Check sheet for the modelled part. Datum: model origin and axes. Units: mm. Face numbers are marked on the shaded views. A direction names the side the tool comes from. Coordinates: 2 decimals unless noted, no trailing zeros. Order: outer loops, then holes, each group sorted by start corner. A loop starts at its lowest first (then second) coordinate and runs counter-clockwise, first axis right, second up.
1. Cross-section at B-B (x = -7.75). Enter the section's corners in (y, z).
2. Thickness scan on line 1 (Y direction, x = -20.45, z = 11.5); line 2 (X direction, y = 1, z = 10) (3 decimals); line 3 (Y direction, x = -13.5, z = 6.75). Record the ranges inside material, lowest first.
3. Set-up check for the marked faces 1, 2, 3, 4 and 5: record each of +Z, -Z, +X, -X, +Y, -Y from which the full face is reachable in a straight line by a thin tool's end or side.
4. Gauge pin test, flat ends, axial feed: pin 1 Ø1.8 at (y, z) = (2.5, 8) entering from +X; pin 2 Ø9 at (y, z) = (-8.5, 13.5) entering from +X; pin 3 Ø3 at (x, y) = (-12.5, -1) entering from -Z; pin 4 Ø1.2 at (y, z) = (3, 3.1) entering from -X. Record the tip position at first contact, or that the pin passes through.
5. Cross-section at C-C (y = 1.25). Enter the section's corners in (x, z), then the cut area to 3 significant figures.
6. Cross-section at D-D (x = -5.5). Enter the section's corners in (y, z).
7. Draft check along X on the marked faces 6, 7, 8 and 9. Enter one of: released by +X, released by -X, zero draft, split by the parting line, or undercut.
8. Cross-section at A-A (z = 10). Enter the section's corners in (x, y).
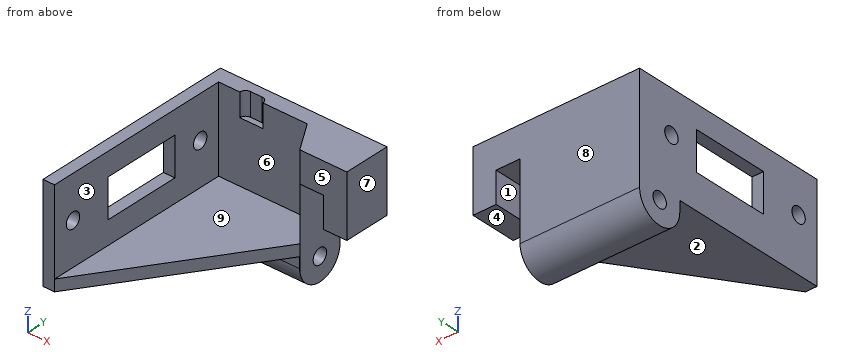
Autodesk Inventor part; units mm, degrees
ref_plane "YZ Plane" through (0, 0, 0) normal (1, 0, 0) x (0, 1, 0)
ref_plane "XZ Plane" through (0, 0, 0) normal (0, 1, 0) x (-1, 0, 0)
ref_plane "XY Plane" through (0, 0, 0) normal (0, 0, 1) x (1, 0, 0)
sketch "Sketch1" plane through (0, 0, 0) normal (0, 1, 0) x (-1, 0, 0)
  line L0 (0, 0) -> (21.6, 0)
  line L1 (21.6, 0) -> (21.6, 17)
  line L2 (21.6, 17) -> (0, 17)
  line L3 (0, 17) -> (0, 0)
  line L4 (6.1, 13) -> (3, 13)
  line L5 (3, 13) -> (3, 0)
  line L6 (3, 0) -> (6.1, 0)
  line L7 (6.1, 0) -> (6.1, 13)
  line L8 (21.6, 17) -> (9.1, 17)
  line L9 (9.1, 17) -> (9.1, 0)
  line L10 (9.1, 0) -> (21.6, 0)
  line L11 (21.6, 0) -> (21.6, 17)
  line L12 (9.1, 17) -> (21.6, 6.2)
  point P0 (21.6, 6.2)
  point P1 (9.1, 17)
  dimension "d1" = 17
  dimension "d2" = 3.1
  dimension "d3" = 3
  dimension "d4" = 3
  dimension "d5" = 6.2
  dimension "d17" = 13
  dimension "d18" = 12.5
extrude "Extrusion1" add sketch "Sketch1" along normal blind 6 contours L3 L2 L9 L0 L7 L4 L5 | L12 L1 L0 L9
sketch "Sketch2" plane through (-21.6, 0, 0) normal (-1, 0, 0) x (0, 0, 1)
  circle A0 centre (3.1, 3) radius 3
  line L0 (0, 0) -> (13, 0)
  line L1 (0, 0) -> (0, 6)
  line L2 (17, 6) -> (0, 6)
  line L3 (0, 0) -> (6.2302, 0)
  line L4 (6.2302, 0) -> (6.2302, 6)
  line L5 (6.2302, 6) -> (0, 6)
  line L6 (0, 6) -> (0, 0)
  circle A1 centre (3.1, 3) radius 1
  point P0 (3.1, 6)
  point P1 (3.1, 0)
  dimension "d8" = 3.1
  dimension "d9" = 2
extrude "Extrusion2" cut sketch "Sketch2" against normal up to surface (18.6 mm away) contours A0 L0 L1 L2 | A1
sketch "Sketch3" plane through (0, 6, 0) normal (0, 1, 0) x (1, 0, 0)
  line L0 (-3, 0) -> (-3, -13)
  line L1 (0, 0) -> (-3, 0)
  line L2 (-3, -9) -> (0, -9)
  line L3 (0, -9) -> (0, 0)
  line L4 (0, 0) -> (-3, 0)
  line L5 (-3, 0) -> (-3, -9)
  line L6 (-3, -13) -> (-6.1, -13)
  line L7 (-9.1, -17) -> (0, -17)
  dimension "d13" = 8
extrude "Extrusion3" cut sketch "Sketch3" against normal blind 10
sketch "Sketch4" plane through (0, 0, 0) normal (0, -1, 0) x (1, 0, 0)
  line L0 (-21.6, 6.2) -> (-9.1, 17)
  line L1 (-9.1, 17) -> (-20.1, 17)
  line L2 (-20.1, 17) -> (-20.1, 7.496)
  line L3 (-20.1, 7.496) -> (-9.1, 7.496)
  line L4 (-9.1, 7.496) -> (-9.1, 17)
  line L5 (-6.1, 13) -> (-6.1, 3.1)
  point P0 (0, 0)
  dimension "d19" = 14
extrude "Extrusion4" cut sketch "Sketch4" against normal blind 4 contours L0 L4 L3
sketch "Sketch5" plane through (0, 0, 0) normal (0, -1, 0) x (1, 0, 0)
  line L0 (-9.1, 17) -> (-9.1, 7.496)
  line L1 (-9.1, 17) -> (-8.6, 17)
  line L2 (-8.6, 17) -> (-8.6, 7.496)
  line L3 (-8.6, 7.496) -> (-9.1, 7.496)
  line L4 (-9.1, 7.496) -> (-9.1, 17)
  line L5 (-6.1, 13) -> (-6.1, 3.1)
  point P0 (0, 0)
  dimension "d22" = 2.5
extrude "Extrusion5" cut sketch "Sketch5" against normal up to surface (4 mm away)
sketch "Sketch7" plane through (0, 4, 0) normal (0, -1, 0) x (1, 0, 0)
  line L0 (-8.6, 7.496) -> (-8.6, 17)
  line L1 (-8.6, 17) -> (-20.1, 17)
  line L2 (-20.1, 17) -> (-20.1, 6)
  line L3 (-20.1, 6) -> (-8.6, 6)
  line L4 (-8.6, 6) -> (-8.6, 17)
  point P0 (0, 0)
  dimension "d25" = 11.5
  dimension "d26" = 11
extrude "Extrusion6" cut sketch "Sketch7" along normal blind 10
sketch "Sketch8" plane through (0, 4, 0) normal (0, -1, 0) x (1, 0, 0)
  line L0 (-20.1, 7.496) -> (-20.1, 6)
  line L1 (-8.6, 6) -> (-8.6, 17)
  line L2 (-20.1, 6) -> (-8.6, 6)
  line L3 (-8.6, 6) -> (-8.6, 17)
  line L4 (-8.6, 17) -> (-20.1, 17)
  line L5 (-20.1, 17) -> (-20.1, 6)
  point P0 (0, 0)
extrude "Extrusion7" add sketch "Sketch8" against normal up to surface (2 mm away)
sketch "Sketch9" plane through (0, 6, 0) normal (0, 1, 0) x (1, 0, 0)
  line L0 (-20.1, -17) -> (-20.1, -7.496)
  line L1 (-21.6, -3.1) -> (-21.6, -6.2)
  line L2 (-20.1, -17) -> (-21.6, -17)
  line L3 (-21.6, -17) -> (-21.6, -6)
  line L4 (-21.6, -6) -> (-20.1, -6)
  line L5 (-20.1, -6) -> (-20.1, -17)
  point P0 (0, 0)
  dimension "d31" = 11
extrude "Extrusion8" add sketch "Sketch9" against normal blind 26.5
sketch "Sketch11" plane through (-20.1, 0, 6) normal (0, 0, -1) x (-1, 0, 0)
  line L0 (0, -20.5) -> (1.5, -20.5)
  line L1 (1.5, -20.5) -> (-13.9653, -20.5)
  line L2 (-13.9653, -20.5) -> (-13.9653, 0)
  line L3 (-13.9653, 0) -> (1.5, 0)
  line L4 (1.5, 0) -> (1.5, -20.5)
  line L5 (-13.9653, 0) -> (0, -20.5)
  point P0 (-20.1, 0)
extrude "Extrusion9" add sketch "Sketch11" along normal blind 2 contours L5 L3 L4 L0
sketch "Sketch13" plane through (-20.1, 4, 17) normal (1, 0, 0) x (0, 0, -1)
  circle A0 centre (5.5, -2.75) radius 1
  circle A1 centre (5.5, -21.75) radius 1
  line L0 (11, -24.5) -> (0, -24.5)
  line L1 (0, 0) -> (11, 0)
  line L2 (8, -6.5185) -> (3, -6.5185)
  line L3 (3, -6.5185) -> (3, -16.5185)
  line L4 (3, -16.5185) -> (8, -16.5185)
  line L5 (8, -16.5185) -> (8, -6.5185)
  line L6 (0, 0) -> (0, -24.5)
  point P0 (17, -4)
  dimension "d36" = 2.75
  dimension "d37" = 2.75
  dimension "d38" = 2
  dimension "d39" = 2
  dimension "d40" = 10
  dimension "d41" = 5
  dimension "d42" = 3
  dimension "d43" = 5.5
  dimension "d44" = 5.5
extrude "Extrusion10" cut sketch "Sketch13" against normal blind 2
chamfer "Chamfer1" distance 2.5 distance2 4 1 edges at (-8.6, 0, 11.5)
sketch "Sketch14" plane through (-20.1, 0, 4) normal (0, 0, -1) x (-1, 0, 0)
  line L0 (1.5, 6) -> (1.5, -20.5)
  line L1 (-14, 6) -> (-14, 0)
  line L2 (1.5, -20.5) -> (-14, -20.5)
  line L3 (-14, -20.5) -> (-14, 0)
  line L4 (-14, 0) -> (1.5, 0)
  line L5 (1.5, 0) -> (1.5, -20.5)
  point P0 (-20.1, 0)
extrude "Extrusion11" cut sketch "Sketch14" against normal blind 0.5
sketch "Sketch15" plane through (-21.6, 6, 17) normal (0, 0, 1) x (1, 0, 0)
  line L0 (1.5, -2) -> (13, -2)
  circle A0 centre (5, -2) radius 0.75
  circle A1 centre (6.5, -2) radius 0.75
  line L1 (5, -2) -> (5.9454, -2)
  line L2 (5, -1.4951) -> (5, -2)
  line L3 (1.5, -2) -> (1.5, -26.5)
  line L4 (5, -2) -> (6.5, -2)
  line L5 (6.5, -2) -> (6.5, -1.25)
  line L6 (6.5, -1.25) -> (5, -1.25)
  line L7 (5, -1.25) -> (5, -2)
  point P0 (21.6, -6)
  point P1 (7.25, -2)
  point P2 (5, -1.25)
  point P3 (4.25, -2)
  dimension "d53" = 1.5
  dimension "d52" = 1.5
  dimension "d54" = 1.5
  dimension "d56" = 0
extrude "Extrusion12" cut sketch "Sketch15" against normal blind 3 contours L2 L7 A0 L0 | L0 A0 L7 L2 | A1 L5 L0 | A0 L6 A1 | A1 L0 L5
properties part number "Pi3B_spacer_R_switch"
Data:
1. outline: (-2.37, 4.5) - (0, 4.5) - (0, 3.1) arc R3 ccw to (6, 3.1) - (6, 17) - (2.64, 17) - (2.64, 6) - (-2.37, 6) - close; hole circle Ø2 at (3, 3.1)
2. line 1: y = -20.5 to -18.75, -16.75 to -12.52, -2.52 to 0.25, 2.25 to 6
2. line 2: x = -21.6 to -20.1, -6.725 to -6.1, -3 to 0
2. line 3: y = 4 to 6
3. face 1: -Z, +Y, -Y
3. face 2: -Z, +X, -X, -Y
3. face 3: +Z, -Y
3. face 4: -Z, +X, +Y, -Y
3. face 5: +Z, -Z, +X, -Y
4. pin 1: stops at x = -6.1
4. pin 2: stops at x = -20.1
4. pin 3: stops at z = 1.44
4. pin 4: passes through
5. outline: (-21.6, 0.66) - (-6.1, 0.66) - (-6.1, 13) - (-3, 13) - (-3, 9) - (0, 9) - (0, 17) - (-6.88, 17) - (-6.88, 6) - (-20.1, 6) - (-20.1, 10.5) - (-21.6, 10.5) - close; (-21.6, 12.5) - (-20.1, 12.5) - (-20.1, 17) - (-21.6, 17) - close
5. area: 141 mm2
6. outline: (0, 13) - (6, 13) - (6, 17) - (0, 17) - close
7. face 6: undercut
7. face 7: released by +X
7. face 8: zero draft
7. face 9: undercut
8. outline: (-21.6, -20.5) - (-20.1, -20.5) - (-20.1, -12.52) - (-21.6, -12.52) - close; (-21.6, -2.52) - (-20.1, -2.52) - (-20.1, 4) - (-8.6, 4) - (-6.1, 0) - (-6.1, 6) - (-21.6, 6) - close; (-3, 0) - (0, 0) - (0, 6) - (-3, 6) - close
